Source: CAD feature listing. Evaluate the final solid. Frame: model axes, mm. A direction names the side the tool comes from. Coordinates: 2 decimals unless noted, no trailing zeros. Order: outer loops, then holes, each group sorted by start corner. A loop starts at its lowest first (then second) coordinate and runs counter-clockwise, first axis right, second up.
Item 1: Section A-A on z = 19.5. Return the cut outline in (x, y), then the cut area to 3 significant figures.
Item 2: Contact query for flat-ended pins moving along their axis: P1, Ø5, axis at y = -16, z = 7, coming from the -X side; P2, Ø12, axis at x = -6.5, y = -1, coming from the -Z side; P3, Ø6, axis at x = 1.5, y = -13, coming from the +Z side; P4, Ø16, axis at x = 3, z = -27.5, coming from the -Y side. Output: stop coordinate, or through.
Item 3: Mould query, pull axis Z, two halves, no side actions, for faces 1 (the flat face through (7, 3, -35.382)), 2 (the cylindrical face through (20.195, 2.535, -23.904)), 3 (the cylindrical face through (20.324, 2.465, 27.425)), 4 (the flat face through (-20.123, -5, 4)). Classes: released by +Z, released by -Z, zero draft, split by the parting line, or undercut.
Item 4: Reachability of faces 5 (the flat face through (-3, 0, 2)), 6 (the flat face through (7, 0, -25)), 7 (the flat face through (-15.123, 2, -25)) from +Z, -Z, +X, -X, +Y, -Y: full face, straight path, thin tool, end or side. Return the list, or none.
Item 5: Section D-D on y = 2.75. Return the cut outline in (x, z), then the cut area to 3 significant figures.
Item 6: Section B-B on x = -12. Return the cut outline in (y, z).
Item 7: Section C-C on z = -4. Return the cut outline in (x, y).
Item 8: Ray query, line 1 (X direction, y = -0.25, z = 11.5); line 2 (Y direction, x = -1, z = -26); line 3 (Z direction, x = 21, y = 2.25). Return the intervals inside material, ascending.
from build123d import *

# Parameters (mm, degrees)
SKETCH_1_W          = 43
SKETCH_1_H          = 43
SKETCH_1_R          = 1.75
SKETCH_1_R_2        = 12.5
EXTRUDE_1_DEPTH     = 5
SKETCH_2_W          = 43
SKETCH_2_H          = 5
EXTRUDE_2_DEPTH     = 25
SKETCH_3_W          = 43
SKETCH_3_H          = 5
EXTRUDE_3_DEPTH     = 20
EXTRUDE_4_DEPTH     = 5
EXTRUDE_6_DEPTH     = 5
SKETCH_10_R         = 2.75
CUT_EXTRUDE_1_DEPTH = 55.385549855


with BuildPart() as part:
    # 草图1 → 凸台-拉伸1 (new body)
    with BuildSketch(Plane(origin=(0, 0, 0), x_dir=(1, 0, 0), z_dir=(0, 1, 0))):
        with Locations((6.376567293, -11.117527558)):
            Rectangle(SKETCH_1_W, SKETCH_1_H)
        with Locations(Location((-9.123432707, -26.617527558, 0), (0, 0, 270))):
            Circle(SKETCH_1_R, mode=Mode.SUBTRACT)
        with Locations(Location((21.876567293, -26.617527558, 0), (0, 0, 270))):
            Circle(SKETCH_1_R, mode=Mode.SUBTRACT)
        with Locations(Location((21.876567293, 4.382472442, 0), (0, 0, 270))):
            Circle(SKETCH_1_R, mode=Mode.SUBTRACT)
        with Locations(Location((-9.123432707, 4.382472442, 0), (0, 0, 270))):
            Circle(SKETCH_1_R, mode=Mode.SUBTRACT)
        with Locations(Location((6.376567293, -11.117527558, 0), (0, 0, 270))):
            Circle(SKETCH_1_R_2, mode=Mode.SUBTRACT)
    extrude(amount=EXTRUDE_1_DEPTH)

    # 草图2 → 凸台-拉伸2 (add)
    with BuildSketch(Plane(origin=(0, 0, -10.382472442), x_dir=(-1, 0, 0), z_dir=(0, 0, -1))):
        with Locations((-6.376567293, 2.5)):
            Rectangle(SKETCH_2_W, SKETCH_2_H)
    extrude(amount=EXTRUDE_2_DEPTH)

    # 草图3 → 凸台-拉伸3 (add)
    with BuildSketch(Plane.XZ):
        with Locations((6.376567293, -12.882472442)):
            Rectangle(SKETCH_3_W, SKETCH_3_H)
    extrude(amount=EXTRUDE_3_DEPTH)

    # 草图4 → 凸台-拉伸4 (add)
    with BuildSketch(Plane(origin=(27.876567293, 0, 0), x_dir=(0, 0, -1), z_dir=(1, 0, 0))):
        Polygon((-32.617527558, 0), (10.382472442, -20), (15.382472442, -20), (15.382472442, 5), (-32.617527558, 5), align=None)
    extrude(amount=EXTRUDE_4_DEPTH)

    # 草图9 → 凸台-拉伸6 (add)
    with BuildSketch(Plane.ZY.offset(15.123432707)):
        Polygon((32.617527558, 5), (32.617527558, 0), (-10.382472442, -20), (-15.382472442, -20), (-15.382472442, 5), align=None)
    extrude(amount=EXTRUDE_6_DEPTH)

    # 草图10 → 切除-拉伸1 (cut, through all)
    with BuildSketch(Plane(origin=(0, 5, 0), x_dir=(1, 0, 0), z_dir=(0, 1, 0))):
        with Locations(Location((-5.123432707, 25.382472442, 0), (0, 0, 270))):
            Circle(SKETCH_10_R)
        with Locations(Location((17.876567293, 25.382472442, 0), (0, 0, 270))):
            Circle(SKETCH_10_R)
    extrude(amount=-CUT_EXTRUDE_1_DEPTH, mode=Mode.SUBTRACT)


solid = part.part
Answer list:
1. outline: (-20.12, -6.1) - (-15.12, -6.1) - (-15.12, 0) - (-2.9, 0) - (-2.9, 5) - (-20.12, 5) - close; (15.65, 0) - (27.88, 0) - (27.88, -6.1) - (32.88, -6.1) - (32.88, 5) - (15.65, 5) - close
1. area: 233 mm2
2. P1: passes through
2. P2: stops at z = -35.38
2. P3: stops at z = -10.38
2. P4: stops at y = 0
3. face 1: released by -Z
3. face 2: undercut
3. face 3: undercut
3. face 4: zero draft
4. face 5: +Z, -Y
4. face 6: -Z, +X, -X, -Y
4. face 7: -Z, -X, +Y, -Y
5. outline: (-20.12, -15.38) - (-15.12, -15.38) - (-15.12, -35.38) - (27.88, -35.38) - (27.88, -15.38) - (32.88, -15.38) - (32.88, 32.62) - (-20.12, 32.62) - close; hole circle Ø3.5 at (-9.12, -4.38); hole circle Ø3.5 at (-9.12, 26.62); hole circle Ø5.5 at (-5.12, -25.38); hole circle Ø25 at (6.38, 11.12); hole circle Ø5.5 at (17.88, -25.38); hole circle Ø3.5 at (21.88, -4.38); hole circle Ø3.5 at (21.88, 26.62)
5. area: 2,830 mm2
6. outline: (-20, -15.38) - (0, -15.38) - (0, -35.38) - (5, -35.38) - (5, 32.62) - (0, 32.62) - (0, -10.38) - (-20, -10.38) - close
7. outline: (-20.12, -17.03) - (-15.12, -17.03) - (-15.12, 0) - (-10.83, 0) - (-10.83, 5) - (-20.12, 5) - close; (-7.42, 0) - (20.17, 0) - (20.17, 5) - (-7.42, 5) - close; (23.58, 0) - (27.88, 0) - (27.88, -17.03) - (32.88, -17.03) - (32.88, 5) - (23.58, 5) - close
8. line 1: x = -20.12 to -15.12, 27.88 to 32.88
8. line 2: y = 0 to 5
8. line 3: z = -35.38 to -5.9, -2.87 to 25.1, 28.13 to 32.62
